Verification items for this drawing (mm, ordinates from the low corner). A direction names the side the tool comes from. Coordinates: 2 decimals unless noted, no trailing zeros. Order: outer loops, then holes, each group sorted by start corner. A loop starts at its lowest first (then second) coordinate and runs counter-clockwise, first axis right, second up. Notation, with made-up numbers: M 51.5,56 L 87.5,56 A29 ccw 87.5,86 Z; hole C 81.5,8 d8. An arc over 180 degrees is marked long. Return JSON: item names as keys, results as strings. Group by question number.
1. Mould release check, pull along X, two halves, no side actions. Record for the marked faces 1, 2, 3 and 4: +X half, -X half, draft (parallel to the pull), parting line (faces both ways), or undercut.
2. Gauge pin test, flat ends, axial feed: pin 1 (8 mm diameter, centred on y = 29, z = 12.5, fed in from -X); pin 2 (7.5 mm diameter, centred on x = 4, z = 12, fed in from -Y); pin 3 (12 mm diameter, centred on x = 92.5, z = 11.5, fed in from +Y); pin 4 (3 mm diameter, centred on y = 29, z = 12.5, fed in from -X). Record the tip position at first contact, or that the pin passes through.
3. Set-up check for the marked faces 5, 6 and 7: record each of +Z, -Z, +X, -X, +Y, -Y from which the full face is reachable in a straight line by a thin tool's end or side.
4. Section check C-C, the plane x = 8.5. Record the cut outline in (y, z).
5. Section check D-D, the plane y = 37. Record the cut outline in (x, z), plus the area to 4 significant figures.
6. Section check A-A, the plane y = 29. Record the cut outline in (x, z), plus the area to 3 significant figures.
7. Material ranges on line 1 along Z through (x, y) = (19, 52); line 2 along Y through (x, z) = (95, 12.5); line 3 along Z through (x, y) = (13.5, 27), recorded low to high.
8. Section check B-B, the plane z = 12.5. Record the cut outline in (x, y).
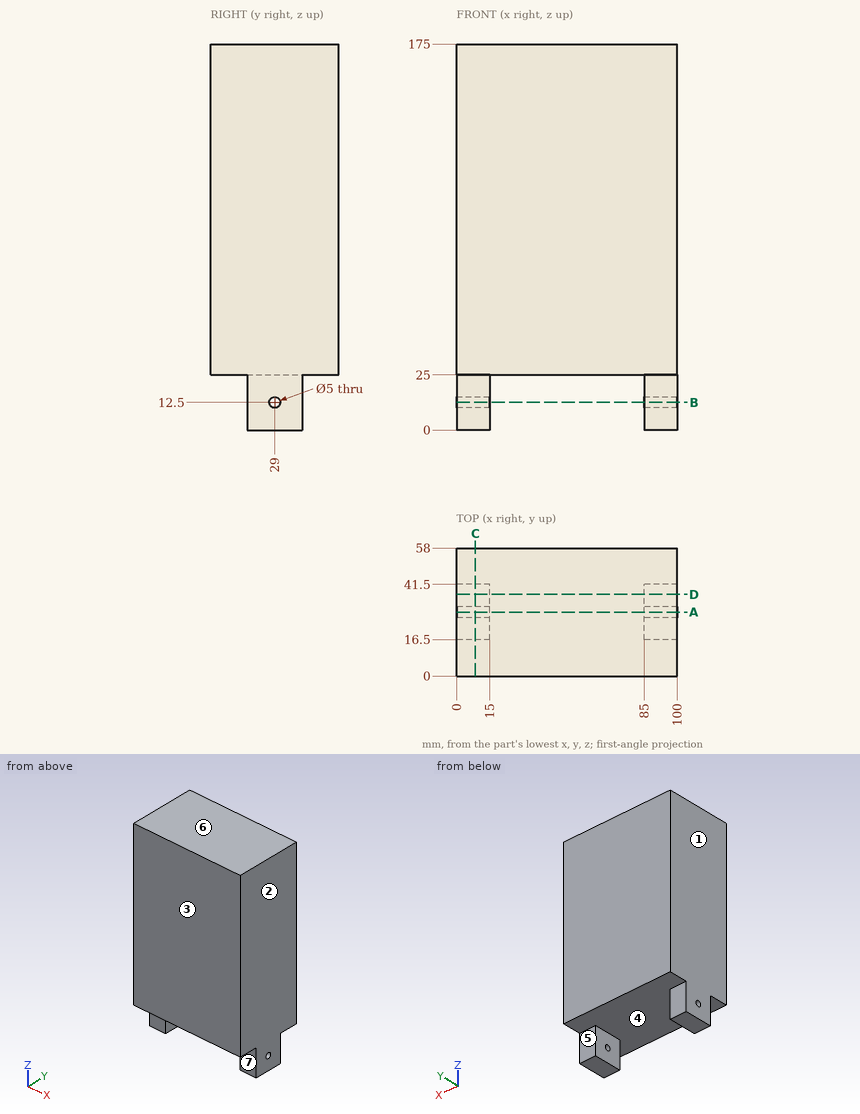
Answers follow:
{
 "1": {"face 1": "-X half", "face 2": "+X half", "face 3": "draft", "face 4": "undercut"},
 "2": {"pin 1": "x = 0", "pin 2": "y = 16.5", "pin 3": "y = 41.5", "pin 4": "through"},
 "3": {"face 5": "-Z, +X, -X, +Y", "face 6": "+Z, +X, -X, +Y, -Y", "face 7": "-Z, +X, -X, -Y"},
 "4": {"outline": "M 0,25 L 16.5,25 L 16.5,0 L 41.5,0 L 41.5,25 L 58,25 L 58,175 L 0,175 Z; hole C 29,12.5 d5"},
 "5": {"outline": "M 0,0 L 15,0 L 15,25 L 85,25 L 85,0 L 100,0 L 100,175 L 0,175 Z", "area": "15,750 mm^2"},
 "6": {"outline": "M 0,0 L 15,0 L 15,10 L 0,10 Z; M 0,15 L 15,15 L 15,25 L 85,25 L 85,15 L 100,15 L 100,175 L 0,175 Z; M 85,0 L 100,0 L 100,10 L 85,10 Z", "area": "15,600 mm^2"},
 "7": {"line 1": "25 to 175", "line 2": "16.5 to 26.5, 31.5 to 41.5", "line 3": "0 to 11, 14 to 175"},
 "8": {"outline": "M 0,16.5 L 15,16.5 L 15,26.5 L 0,26.5 Z; M 0,31.5 L 15,31.5 L 15,41.5 L 0,41.5 Z; M 85,16.5 L 100,16.5 L 100,26.5 L 85,26.5 Z; M 85,31.5 L 100,31.5 L 100,41.5 L 85,41.5 Z"}
}
